The figure shows three views and two pictorial views of one solid part (mm, origin at its lowest corner). Answer the questions. A direction names the side the tool comes from. Give positions to 0.01 mm unless a question says otherwise; leave off trailing zeros. Loops run counter-clockwise (first coordinate to the right, second up) from the corner with the lowest first, then second, coordinate; pieces in that order, holes last. Notation, with made-up numbers: (19, -27) - (70, -27) arc R26 ccw to (70, -10) - close; hole circle Ø2 at (36, 20.25). An arc over 180 degrees is marked (long way). One line per question, with ' | ' between items.
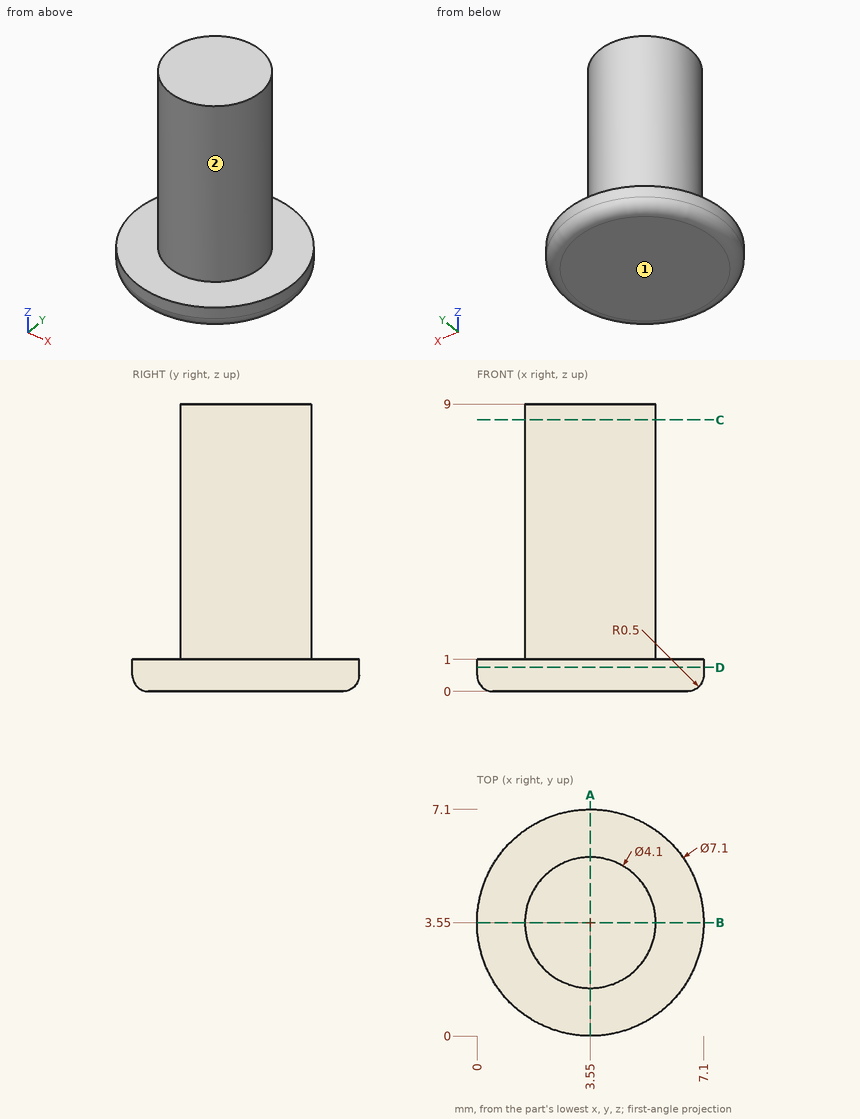
1. Consider L1, parallel to Y at x = 3.5, z = 5.5; L2, parallel to Z at x = 5, y = 6.25; L3, parallel to X at y = 5, z = 0.5. Determine where each line is inside the solid, lowest interval first.
Evaluation:
L1: 1.5 to 5.6 | L2: 0 to 1 | L3: 0.31 to 6.79
2. Find section A-A on x = 3.55. Write down the section's boundary in (y, z), then the cut area to 3 significant figures.
Evaluation:
outline: (0, 0.5) arc R0.5 ccw to (0.5, 0) - (6.6, 0) arc R0.5 ccw to (7.1, 0.5) - (7.1, 1) - (5.6, 1) - (5.6, 9) - (1.5, 9) - (1.5, 1) - (0, 1) - close | area: 39.8 mm2
3. Flat-ended cylindrical pins translate along their axes: pin 1 (1 mm diameter, centred on x = 5, y = 1.5, fed in from +Z); pin 2 (1.5 mm diameter, centred on x = 2.5, z = 5, fed in from +Y). Find the tip coordinate at first contact, or state that the pin passes through.
Evaluation:
pin 1: z = 9 | pin 2: y = 5.58
4. Which of the six approach directions +Z, -Z, +X, -X, +Y, -Y give full straight-line access (tool end or side, diameter ignored) to the marked faces 1 and 2?
Evaluation:
face 1: -Z, +X, -X, +Y, -Y | face 2: +Z
5. Find section C-C on z = 8.5. Write down the section's boundary in (x, y).
Evaluation:
outline: circle Ø4.1 at (3.55, 3.55)
6. Find section D-D on z = 0.75. Write down the section's boundary in (x, y), then the cut area to 3 significant figures.
Evaluation:
outline: circle Ø7.1 at (3.55, 3.55) | area: 39.6 mm2
